```python
from build123d import *

# Parameters (mm, degrees)
SKETCH1_R           = 2
BOSS_EXTRUDE1_DEPTH = 3


with BuildPart() as part:
    # Sketch1 → Boss-Extrude1 (new body)
    with BuildSketch(Plane.XY):
        with BuildLine():
            Line((-50, 48), (50, 48))
            ThreePointArc((50, 48), (57.071067812, 45.071067812), (60, 38))
            Line((60, 38), (60, -38))
            ThreePointArc((60, -38), (57.071067812, -45.071067812), (50, -48))
            Line((50, -48), (-50, -48))
            ThreePointArc((-50, -48), (-57.071067812, -45.071067812), (-60, -38))
            Line((-60, -38), (-60, 38))
            ThreePointArc((-60, 38), (-57.071067812, 45.071067812), (-50, 48))
        make_face()
        with Locations((0, 32)):
            Circle(SKETCH1_R, mode=Mode.SUBTRACT)
        with Locations((0, -32)):
            Circle(SKETCH1_R, mode=Mode.SUBTRACT)
        with Locations((32, 0)):
            Circle(SKETCH1_R, mode=Mode.SUBTRACT)
        with Locations((-32, 0)):
            Circle(SKETCH1_R, mode=Mode.SUBTRACT)
        with Locations((-50, 38)):
            Circle(SKETCH1_R, mode=Mode.SUBTRACT)
        with Locations((50, 38)):
            Circle(SKETCH1_R, mode=Mode.SUBTRACT)
        with Locations((50, -38)):
            Circle(SKETCH1_R, mode=Mode.SUBTRACT)
        with Locations((-50, -38)):
            Circle(SKETCH1_R, mode=Mode.SUBTRACT)
        with Locations((-38, -27.5)):
            Circle(SKETCH1_R, mode=Mode.SUBTRACT)
        with Locations((38, -27.5)):
            Circle(SKETCH1_R, mode=Mode.SUBTRACT)
        with Locations((0, -41)):
            Circle(SKETCH1_R, mode=Mode.SUBTRACT)
        with BuildLine():
            Line((17.35191045, -35), (32.64808955, -35))
            ThreePointArc((32.64808955, -35), (35.64808955, -38), (32.64808955, -41))
            Line((32.64808955, -41), (17.35191045, -41))
            ThreePointArc((17.35191045, -41), (14.35191045, -38), (17.35191045, -35))
        make_face(mode=Mode.SUBTRACT)
        with BuildLine():
            Line((52.5, 25), (52.5, -25))
            ThreePointArc((52.5, -25), (50, -27.5), (47.5, -25))
            Line((47.5, -25), (47.5, 25))
            ThreePointArc((47.5, 25), (50, 27.5), (52.5, 25))
        make_face(mode=Mode.SUBTRACT)
        with BuildLine():
            Line((-47.5, 25), (-47.5, -25))
            ThreePointArc((-47.5, -25), (-50, -27.5), (-52.5, -25))
            Line((-52.5, -25), (-52.5, 25))
            ThreePointArc((-52.5, 25), (-50, 27.5), (-47.5, 25))
        make_face(mode=Mode.SUBTRACT)
        with BuildLine():
            Line((-32.64808955, -35), (-17.35191045, -35))
            ThreePointArc((-17.35191045, -35), (-14.35191045, -38), (-17.35191045, -41))
            Line((-17.35191045, -41), (-32.64808955, -41))
            ThreePointArc((-32.64808955, -41), (-35.64808955, -38), (-32.64808955, -35))
        make_face(mode=Mode.SUBTRACT)
    extrude(amount=BOSS_EXTRUDE1_DEPTH)


solid = part.part
```
Build history of the part. All positions in model axes, mm. A direction names the side the tool comes from. Round coordinates to 2 decimals unless told otherwise and drop trailing zeros. Write each loop counter-clockwise with the first axis right and the second up, starting at its lowest first coordinate (ties: lowest second). Pieces come first, ordered by that corner, then holes.
1) Pin check, flat tip, straight feed: pin 1 (6 mm diameter, centred on x = -42.5, y = -16.5, fed in from -Z). Stop position of the tip, or through.
2) Band-saw the part on B-B, the plane x = 27. List the corners of the cut face in (y, z).
3) Mould opens along Y. For faces 3 (the cylindrical face through (-57.15, 44.99, 1.48)), 4 (the flat face through (1, -48, 1)), 5 (the flat face through (-52.5, 0, 1)), 6 (the flat face through (25, -35, 1)) say: +Y half, -Y half, draft (parallel to the pull), parting line (faces both ways), or undercut.
4) 3-axis set-ups, long thin cutter, end or side, ignore diameter. For faces 1 (the flat face through (-25, -41, 1)), 2 (the flat face through (1, 1, 0)): which of +Z, -Z, +X, -X, +Y, -Y reach the whole face in a straight line?
5) Band-saw the part on C-C, the plane y = -5. List the corners of the cut face in (x, z), and give its area (3 significant figures).
6) Drill centre lines: probe 1 along Y at (x, z) = (32, 1.9); probe 2 along Y at (x, z) = (0, 0.8); probe 3 along X at (y, z) = (9, 2.55). Where is each one in solid material? Low to high.
7) Band-saw the part on A-A, the plane y = -32. List the corners of the cut face in (x, z).
8) Band-saw the part on D-D, the plane z = 1.2. Give the number of separate pieces and of enclosed holes in the cut face, and give its area (3 significant figures).
Ans:
1. pin 1: stops at z = 0
2. outline: (-48, 0) - (-41, 0) - (-41, 3) - (-48, 3) - close; (-35, 0) - (48, 0) - (48, 3) - (-35, 3) - close
3. face 3: +Y half
3. face 4: -Y half
3. face 5: undercut
3. face 6: undercut
4. face 1: +Z, -Z
4. face 2: -Z, +X, -X, +Y, -Y
5. outline: (-60, 0) - (-52.5, 0) - (-52.5, 3) - (-60, 3) - close; (-47.5, 0) - (47.5, 0) - (47.5, 3) - (-47.5, 3) - close; (52.5, 0) - (60, 0) - (60, 3) - (52.5, 3) - close
5. area: 330 mm2
6. probe 1: y = -48 to -41, -35 to -2, 2 to 48
6. probe 2: y = -48 to -43, -39 to -34, -30 to 30, 34 to 48
6. probe 3: x = -60 to -52.5, -47.5 to 47.5, 52.5 to 60
7. outline: (-60, 0) - (-2, 0) - (-2, 3) - (-60, 3) - close; (2, 0) - (60, 0) - (60, 3) - (2, 3) - close
8. separate pieces: 1
8. enclosed holes: 15
8. area: 10,500 mm2
